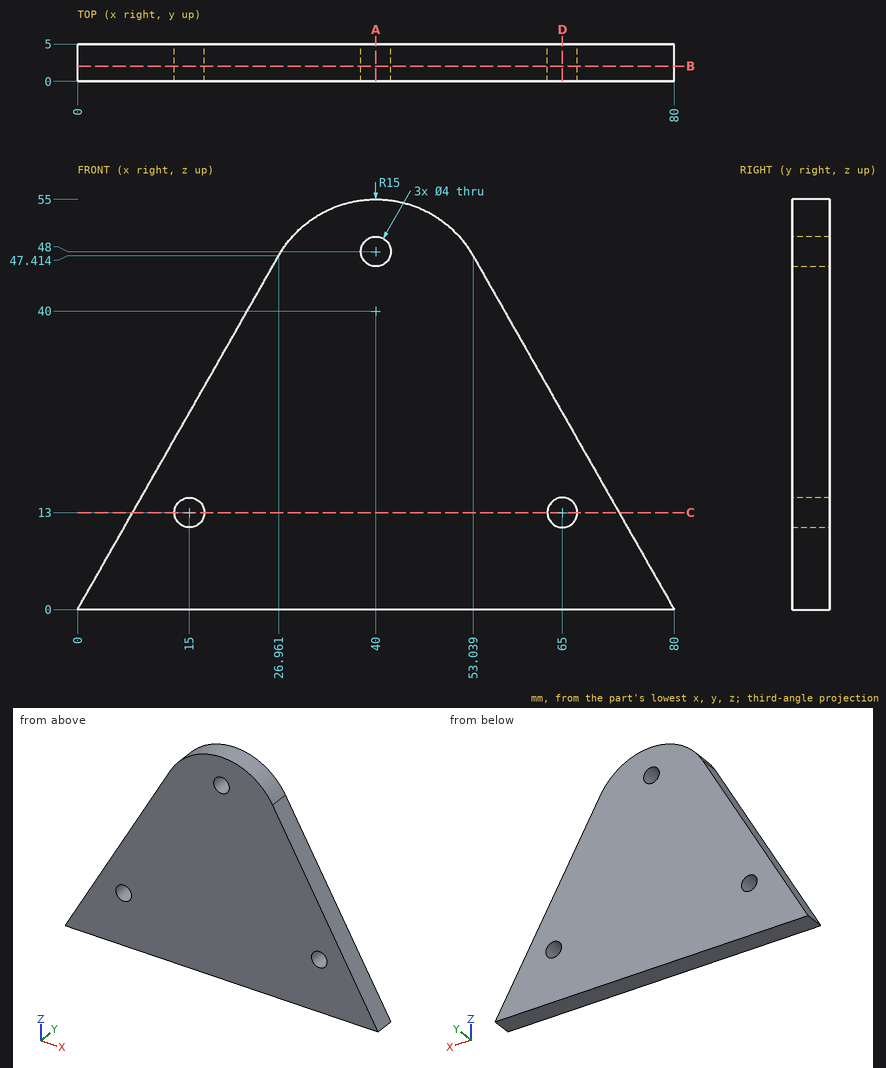
Verification items for this drawing (mm, ordinates from the low corner). Give positions to 0.01 mm unless a question says otherwise; leave off trailing zeros. Loops run counter-clockwise (first coordinate to the right, second up) from the corner with the lowest first, then second, coordinate; pieces in that order, holes last. Notation, with made-up numbers: M 81,0.25 L 117,0.25 A20 cw 117,21.25 Z; hole C 89,-38.5 d11. An arc over 180 degrees is marked long. Answer as a JSON object with one key per item and string values. Group by question number.
Item 1: Sectioned sample at A-A on x = 40. Record the boundary of the cut face in (y, z).
Item 2: Gauge pin test, flat end, axial feed: pin 1 (2 mm diameter, centred on y = 0.5, z = 8, fed in from +X). Record the tip position at first contact, or that the pin passes through.
Item 3: Material ranges on L1, parallel to X at y = 1.95, z = 13; L2, parallel to Z at x = 65, y = 1.6; L3, parallel to Z at x = 65.5, y = 3.1 (1 decimal), recorded low to high.
Item 4: Sectioned sample at C-C on z = 13. Record the boundary of the cut face in (x, y).
Item 5: Sectioned sample at B-B on y = 2.05. Record the boundary of the cut face in (x, z) (1 decimal), plus the area to 3 significant figures.
Item 6: Sectioned sample at D-D on x = 65. Record the boundary of the cut face in (y, z).
Findings below:
{
 "1": {"outline": "M 0,0 L 5,0 L 5,46 L 0,46 Z; M 0,50 L 5,50 L 5,55 L 0,55 Z"},
 "2": {"pin 1": "x = 76.02"},
 "3": {"L1": "7.39 to 13, 17 to 63, 67 to 72.61", "L2": "0 to 11, 15 to 26.38", "L3": "0 to 11.1, 14.9 to 25.5"},
 "4": {"outline": "M 7.39,0 L 13,0 L 13,5 L 7.39,5 Z; M 17,0 L 63,0 L 63,5 L 17,5 Z; M 67,0 L 72.61,0 L 72.61,5 L 67,5 Z"},
 "5": {"outline": "M 0,0 L 80,0 L 53,47.4 A15 ccw 27,47.4 Z; hole C 15,13 d4; hole C 40,48 d4; hole C 65,13 d4", "area": "2,620 mm2"},
 "6": {"outline": "M 0,0 L 5,0 L 5,11 L 0,11 Z; M 0,15 L 5,15 L 5,26.38 L 0,26.38 Z"}
}
